```python
from build123d import *

# Parameters (mm, degrees)
SKETCH1_R           = 1.449927
SKETCH1_R_2         = 1.449937953
SKETCH1_R_3         = 0.874912417
SKETCH1_R_4         = 2.499893062
SKETCH1_RX          = 9.072899251
SKETCH1_RY          = 7.568087766
SKETCH1_RX_2        = 8.777378771
SKETCH1_RY_2        = 5.601336902
SKETCH1_W           = 6.19999
SKETCH1_H           = 3.400011
BOSS_EXTRUDE3_DEPTH = 5.85


with BuildPart() as part:
    # Sketch1 → Boss-Extrude3 (new body)
    with BuildSketch(Plane.XY):
        with BuildLine():
            ThreePointArc((586.387462743, 493.254803119), (611.911693149, 450.352706702), (586.387462742, 407.450610286))
            ThreePointArc((586.387462742, 407.450610286), (584.387859448, 402.590740006), (586.410373629, 397.740359727))
            ThreePointArc((586.410373629, 397.740359727), (586.433284516, 388.030109168), (596.143535075, 388.053020055))
            ThreePointArc((596.143535075, 388.053020055), (601.003405354, 386.053416761), (605.853785634, 388.075930942))
            ThreePointArc((605.853785634, 388.075930942), (648.462479749, 416.506624656), (691.071173865, 388.075930942))
            ThreePointArc((691.071173865, 388.075930942), (695.921554144, 386.053416761), (700.781424424, 388.053020055))
            ThreePointArc((700.781424424, 388.053020055), (710.491674982, 388.030109168), (710.514585869, 397.740359727))
            ThreePointArc((710.514585869, 397.740359727), (712.53710005, 402.590740006), (710.537496756, 407.450610285))
            ThreePointArc((710.537496756, 407.450610285), (685.01326635, 450.352706702), (710.537496756, 493.254803119))
            ThreePointArc((710.537496756, 493.254803119), (712.53710005, 498.114673398), (710.514585869, 502.965053678))
            ThreePointArc((710.514585869, 502.965053678), (710.491674982, 512.675304236), (700.781424424, 512.652393349))
            ThreePointArc((700.781424424, 512.652393349), (695.921554144, 514.651996644), (691.071173865, 512.629482462))
            ThreePointArc((691.071173865, 512.629482462), (648.462479749, 484.198788748), (605.853785634, 512.629482462))
            ThreePointArc((605.853785634, 512.629482462), (601.003405354, 514.651996644), (596.143535075, 512.652393349))
            ThreePointArc((596.143535075, 512.652393349), (586.433284516, 512.675304236), (586.41037363, 502.965053678))
            ThreePointArc((586.41037363, 502.965053678), (584.387859448, 498.114673398), (586.387462743, 493.254803119))
        make_face()
        with Locations((648.462479749, 478.880494)):
            Circle(SKETCH1_R, mode=Mode.SUBTRACT)
        with Locations((682.660917541, 462.166264459)):
            Circle(SKETCH1_R_2, mode=Mode.SUBTRACT)
        with Locations((600.964294024, 498.075562068)):
            Circle(SKETCH1_R_3, mode=Mode.SUBTRACT)
        with Locations((591.254043465, 498.098472955)):
            Circle(SKETCH1_R_3, mode=Mode.SUBTRACT)
        with Locations((591.276954352, 507.808723514)):
            Circle(SKETCH1_R_3, mode=Mode.SUBTRACT)
        with Locations((600.987204911, 507.785812627)):
            Circle(SKETCH1_R_3, mode=Mode.SUBTRACT)
        with Locations((596.120624188, 502.942142791)):
            Circle(SKETCH1_R_4, mode=Mode.SUBTRACT)
        with Locations((700.804335311, 502.942142791)):
            Circle(SKETCH1_R_4, mode=Mode.SUBTRACT)
        with Locations((695.937754588, 507.785812627)):
            Circle(SKETCH1_R_3, mode=Mode.SUBTRACT)
        with Locations((705.648005146, 507.808723514)):
            Circle(SKETCH1_R_3, mode=Mode.SUBTRACT)
        with Locations((705.670916033, 498.098472955)):
            Circle(SKETCH1_R_3, mode=Mode.SUBTRACT)
        with Locations((695.960665475, 498.075562068)):
            Circle(SKETCH1_R_3, mode=Mode.SUBTRACT)
        with Locations((614.264041957, 462.166264459)):
            Circle(SKETCH1_R_2, mode=Mode.SUBTRACT)
        with Locations((614.264041957, 438.539148946)):
            Circle(SKETCH1_R_2, mode=Mode.SUBTRACT)
        with Locations((695.960665475, 402.629851336)):
            Circle(SKETCH1_R_3, mode=Mode.SUBTRACT)
        with Locations((705.670916033, 402.606940449)):
            Circle(SKETCH1_R_3, mode=Mode.SUBTRACT)
        with Locations((705.648005146, 392.896689891)):
            Circle(SKETCH1_R_3, mode=Mode.SUBTRACT)
        with Locations((695.937754588, 392.919600778)):
            Circle(SKETCH1_R_3, mode=Mode.SUBTRACT)
        with Locations((700.804335311, 397.763270613)):
            Circle(SKETCH1_R_4, mode=Mode.SUBTRACT)
        with Locations((596.120624188, 397.763270613)):
            Circle(SKETCH1_R_4, mode=Mode.SUBTRACT)
        with Locations((600.987204911, 392.919600778)):
            Circle(SKETCH1_R_3, mode=Mode.SUBTRACT)
        with Locations((591.276954352, 392.896689891)):
            Circle(SKETCH1_R_3, mode=Mode.SUBTRACT)
        with Locations((591.254043465, 402.606940449)):
            Circle(SKETCH1_R_3, mode=Mode.SUBTRACT)
        with Locations((600.964294024, 402.629851336)):
            Circle(SKETCH1_R_3, mode=Mode.SUBTRACT)
        with Locations((682.660917541, 438.539148946)):
            Circle(SKETCH1_R_2, mode=Mode.SUBTRACT)
        with Locations((648.462479749, 421.824919404)):
            Circle(SKETCH1_R, mode=Mode.SUBTRACT)
        with Locations((608.496752749, 490.507474302)):
            Ellipse(SKETCH1_RX, SKETCH1_RY, mode=Mode.SUBTRACT)
        with Locations(Location((670.798820229, 481.426311828), (0, 0, 180))):
            Ellipse(SKETCH1_RX_2, SKETCH1_RY_2, mode=Mode.SUBTRACT)
        with Locations(Location((688.428206749, 490.507474302), (0, 0, 180))):
            Ellipse(SKETCH1_RX, SKETCH1_RY, mode=Mode.SUBTRACT)
        with Locations((626.12613927, 481.426311828)):
            Ellipse(SKETCH1_RX_2, SKETCH1_RY_2, mode=Mode.SUBTRACT)
        with Locations((626.12613927, 419.279101576)):
            Ellipse(SKETCH1_RX_2, SKETCH1_RY_2, mode=Mode.SUBTRACT)
        with Locations(Location((688.428206749, 410.197939102), (0, 0, 180))):
            Ellipse(SKETCH1_RX, SKETCH1_RY, mode=Mode.SUBTRACT)
        with Locations(Location((670.798820229, 419.279101576), (0, 0, 180))):
            Ellipse(SKETCH1_RX_2, SKETCH1_RY_2, mode=Mode.SUBTRACT)
        with Locations((608.496752749, 410.197939102)):
            Ellipse(SKETCH1_RX, SKETCH1_RY, mode=Mode.SUBTRACT)
        with Locations((614.248765499, 473.5132475)):
            Rectangle(SKETCH1_W, SKETCH1_H, mode=Mode.SUBTRACT)
        with Locations((682.676194, 473.5132475)):
            Rectangle(SKETCH1_W, SKETCH1_H, mode=Mode.SUBTRACT)
        with Locations((682.676194, 427.192165904)):
            Rectangle(SKETCH1_W, SKETCH1_H, mode=Mode.SUBTRACT)
        with Locations((614.248765499, 427.192165904)):
            Rectangle(SKETCH1_W, SKETCH1_H, mode=Mode.SUBTRACT)
        with BuildLine():
            ThreePointArc((652.62969556, 480.08666297), (671.118523525, 470.054927983), (678.48703375, 450.352706702))
            ThreePointArc((678.48703375, 450.352706702), (671.118523525, 430.650485421), (652.62969556, 420.618750434))
            ThreePointArc((652.62969556, 420.618750434), (651.520237389, 423.763672389), (648.462479749, 425.094668164))
            ThreePointArc((648.462479749, 425.094668164), (645.40472211, 423.763672389), (644.295263939, 420.618750434))
            ThreePointArc((644.295263939, 420.618750434), (625.806435974, 430.650485421), (618.437925749, 450.352706702))
            ThreePointArc((618.437925749, 450.352706702), (625.806435974, 470.054927983), (644.295263939, 480.08666297))
            ThreePointArc((644.295263939, 480.08666297), (645.40472211, 476.941741015), (648.462479749, 475.610745241))
            ThreePointArc((648.462479749, 475.610745241), (651.520237389, 476.941741015), (652.62969556, 480.08666297))
        make_face(mode=Mode.SUBTRACT)
    extrude(amount=BOSS_EXTRUDE3_DEPTH)


solid = part.part
```
Build history of the part. All positions in model axes, mm. A direction names the side the tool comes from. Coordinates: 2 decimals unless noted, no trailing zeros. Order: outer loops, then holes, each group sorted by start corner. A loop starts at its lowest first (then second) coordinate and runs counter-clockwise, first axis right, second up. Notation, with made-up numbers: (38.25, -0.75) -> (67.25, -0.75) arc R23 cw to (67.25, 38.25) -> close; hole circle Ø11 at (72, -8). An arc over 180 degrees is marked (long way). Answer in a Markdown table with one row per item. Add a question column.
Q1. Which spindle directions (+Z, -Z, +X, -X, +Y, -Y) get a long thin tool onto all of the face, cutting with end or side? Do faces 3 (the face through (695.846, 386.054, 2.884)), 4 (the face through (683, 425.492, 3)). Say none if no direction does.
Q2. Drop flat-ended pins along their axis: pin 1 (12 mm diameter, centred on x = 600.5, y = 454.5, fed in from -Z); pin 2 (2 mm diameter, centred on x = 672.5, z = 3, fed in from +Y); pin 3 (2.5 mm diameter, centred on y = 474, z = 4, fed in from +X); pin 4 (1.8 mm diameter, centred on x = 613.5, z = 2, fed in from -Y). Give the stop position or say it passes through.
Q3. Wall check: line 1 along Y through (x, z) = (671.5, 4.2); line 2 along X through (y, z) = (423, 4.05); line 3 along Y through (x, z) = (706, 2.8). Give the ranges that are in metal, low to high. Write a range as [from, to].
Q4. Band-saw the part on B-B, the plane x = 638. List the corners of the cut face in (y, z), then the cut area to 3 significant figures.
Q5. Mould opens along X. For faces 1 (the face through (712.537, 498.039, 2.884)), 2 (the face through (586.54, 512.78, 2.88)) say: +X half, -X half, draft (parallel to the pull), parting line (faces both ways), or undercut.
Q6. Band-saw the part on C-C, the plane x = 689.5. Give the number of separate pieces and of enclosed holes in the cut face, then the cut area to 3 significant figures.
Q7. Band-saw the part on A-A, the plane y = 469. List the corners of the cut face in (x, z), then the cut area to 3 significant figures.
Answers follow:
| question | item | result |
|---|---|---|
| 1 | face 3 | +Z, -Z, -Y |
| 1 | face 4 | +Z, -Z |
| 2 | pin 1 | through |
| 2 | pin 2 | y = 491.58 |
| 2 | pin 3 | x = 691.84 |
| 2 | pin 4 | y = 399.4 |
| 3 | line 1 | [410.34, 413.7], [424.86, 431.1], [469.61, 475.84], [487.01, 490.36] |
| 3 | line 2 | [603.53, 619.57], [632.69, 636.08], [644.84, 647.61], [649.31, 652.08], [660.84, 664.24], [677.36, 693.4] |
| 3 | line 3 | [386.04, 392.1], [393.7, 401.8], [403.42, 410.25], [490.46, 497.29], [498.91, 507.01], [508.61, 514.67] |
| 4 | outline | (415.3, 0) -> (422.21, 0) -> (422.21, 5.85) -> (415.3, 5.85) -> close; (478.5, 0) -> (485.4, 0) -> (485.4, 5.85) -> (478.5, 5.85) -> close |
| 4 | area | 80.8 mm^2 |
| 5 | face 1 | +X half |
| 5 | face 2 | undercut |
| 6 | separate pieces | 4 |
| 6 | enclosed holes | 0 |
| 6 | area | 274 mm^2 |
| 7 | outline | (608.21, 0) -> (624.93, 0) -> (624.93, 5.85) -> (608.21, 5.85) -> close; (671.99, 0) -> (688.72, 0) -> (688.72, 5.85) -> (671.99, 5.85) -> close |
| 7 | area | 196 mm^2 |
